Read the model definition and answer for the solid it produces. Units are mm, in the model's axes. Face numbers are marked on the shaded views. A direction names the side the tool comes from. Give positions to 0.01 mm unless a question says otherwise; leave off trailing zeros. Order: outer loops, then holes, each group sorted by start corner. A loop starts at its lowest first (then second) coordinate and runs counter-clockwise, first axis right, second up. Notation, with made-up numbers: (-2, -33.5) -> (11, -33.5) arc R20 ccw to (11, -5.5) -> close; hole circle Ø9 at (56.25, -22.5). An arc over 180 degrees is marked (long way). One line per question, with ' | ' between items. Start each with the question number.
```python
from build123d import *

# Parameters (mm, degrees)
F0_W     = 431.8
F0_H     = 615
F1_DEPTH = 1.5
F2_W     = 615
F2_H     = 173.5
F3_DEPTH = 1.5
F4_W     = 615
F4_H     = 173.5
F5_DEPTH = 1.5
F6_R     = 1.5
F8_D     = 6.7564
F9_D     = 3.3


with BuildPart() as f1:
    # F0 (on Top) → F1 (new body)
    with BuildSketch(Plane.XY):
        Rectangle(F0_W, F0_H)
    extrude(amount=-F1_DEPTH)

    # F2 (on face) → F3 (join)
    with BuildSketch(Plane(origin=(-215.9, 0, 0), x_dir=(0, -1, 0), z_dir=(-1, 0, 0))):
        with Locations((0, 86.75)):
            Rectangle(F2_W, F2_H)
    extrude(amount=-F3_DEPTH)

    # F4 (on face) → F5 (join)
    with BuildSketch(Plane.YZ.offset(215.9)):
        with Locations((0, 86.75)):
            Rectangle(F4_W, F4_H)
    extrude(amount=-F5_DEPTH)

    # F6
    f6_edges = [f1.edges().sort_by_distance(p)[0] for p in [
        (-215.9, 0, -1.5),
        (215.9, 0, -1.5),
    ]]
    fillet(f6_edges, radius=F6_R)

    # F8 (through all)
    with Locations(Plane(origin=(0, 0, -1.5), x_dir=(1, 0, 0), z_dir=(0, 0, -1))):
        with Locations((-84.1375, 143.35), (-17.4625, 143.35), (49.2125, 143.35), (115.8875, 143.35), (182.5625, 143.35), (182.5625, -196.375), (115.8875, -196.375), (49.2125, -196.375), (-17.4625, -196.375), (-84.1375, -196.375), (-150.8125, -196.375), (-150.8125, 143.35)):
            Hole(F8_D / 2)

    # F9 (through all)
    with Locations(Plane(origin=(0, 0, -1.5), x_dir=(1, 0, 0), z_dir=(0, 0, -1))):
        with Locations((-33.382, 267.5), (88.618, 267.5)):
            Hole(F9_D / 2)


solid = f1.part
```
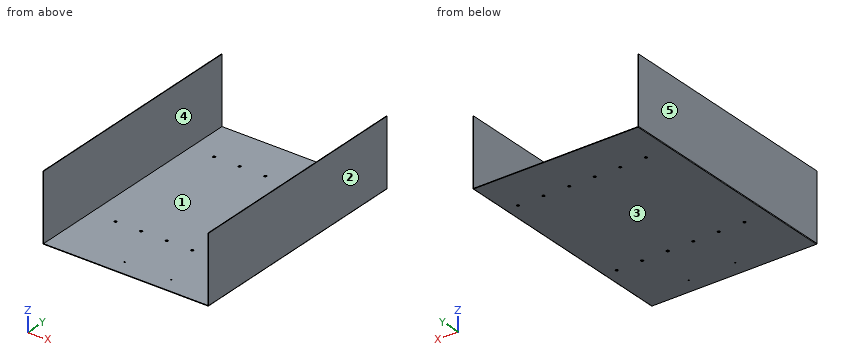
Q1. A cutting plane is placed at A-A, the plane z = 64.5. Determine the outline of the cut face in (x, y).
Q2. Which of the six approach directions +Z, -Z, +X, -X, +Y, -Y give full straight-line access (tool end or side, diameter ignored) to the marked faces 4 and 5?
Q3. A cutting plane is placed at B-B, the plane y = 37.5. Determine the outline of the cut face in (x, z), then the cut area to 3 significant figures.
Q4. Determine the mould class of the marked faces 1, 2 and 3 for opening direction X: pulls with the +X half, pulls with the -X half, needs draft (parallel to the pull), parting line crosses it, or undercut.
Q5. Find the intervals of material crossed by line 1 (X direction, y = -267.5, z = -0.55); line 2 (X direction, y = 282, z = 17.5); line 3 (Z direction, x = 164, y = 142.5), in increasing order.
Q6. Given P1, Ø9, axis at x = -150.81, y = 196.38, coming from the -Z side; P2, Ø4, axis at x = -167.5, y = -25, coming from the +Z side, each flat-ended and moving along its own axis, determine where each tip first touches the part or whether it passes through.
Geometry results:
1) outline: (-215.9, -307.5) -> (-214.4, -307.5) -> (-214.4, 307.5) -> (-215.9, 307.5) -> close; (214.4, -307.5) -> (215.9, -307.5) -> (215.9, 307.5) -> (214.4, 307.5) -> close
2) face 4: +Z, +Y, -Y | face 5: +Z, -Z, -X, +Y, -Y
3) outline: (-215.9, 0) arc R1.5 ccw to (-214.4, -1.5) -> (214.4, -1.5) arc R1.5 ccw to (215.9, 0) -> (215.9, 173.5) -> (214.4, 173.5) -> (214.4, 0) -> (-214.4, 0) -> (-214.4, 173.5) -> (-215.9, 173.5) -> close | area: 1,170 mm²
4) face 1: undercut | face 2: pulls with the +X half | face 3: needs draft
5) line 1: -215.8 to -35.03, -31.73 to 86.97, 90.27 to 215.8 | line 2: -215.9 to -214.4, 214.4 to 215.9 | line 3: -1.5 to 0
6) P1: z = -1.5 | P2: z = 0
